Build history of the part. All positions in model axes, mm. A direction names the side the tool comes from. Give positions to 0.01 mm unless a question says otherwise; leave off trailing zeros. Order: outer loops, then holes, each group sorted by start corner. A loop starts at its lowest first (then second) coordinate and runs counter-clockwise, first axis right, second up. Notation, with made-up numbers: M 22.5,0.5 L 69.5,0.5 A17 ccw 69.5,8.5 Z; hole C 86.5,-35 d2. An arc over 180 degrees is marked long. Answer as CSV lines item,"result".
from build123d import *

# Parameters (mm, degrees)
SKETCH_1_R      = 1.75
SKETCH_1_W      = 65.5
SKETCH_1_H      = 80
EXTRUDE_1_DEPTH = 1
FILLET_1_R      = 1
FILLET_2_R      = 2


with BuildPart() as part:
    # 草圖1 → 填料-伸長1 (new body)
    with BuildSketch(Plane.XY):
        Polygon((-35.75, -20.56252042), (-43, -20.56252042), (-43, -50), (-25.75, -50), (25.75, -50), (43, -50), (43, -20.56252042), (35.75, -20.56252042), (35.75, 20.56252042), (43, 20.56252042), (43, 50), (25.75, 50), (-25.75, 50), (-43, 50), (-43, 20.56252042), (-35.75, 20.56252042), align=None)
        with Locations((-40, -26)):
            Circle(SKETCH_1_R, mode=Mode.SUBTRACT)
        with Locations(Location((40, -26, 0), (0, 0, 180))):
            Circle(SKETCH_1_R, mode=Mode.SUBTRACT)
        with Locations((40, 26)):
            Circle(SKETCH_1_R, mode=Mode.SUBTRACT)
        with Locations(Location((-40, 26, 0), (0, 0, 180))):
            Circle(SKETCH_1_R, mode=Mode.SUBTRACT)
        with Locations((-40, -46)):
            Circle(SKETCH_1_R, mode=Mode.SUBTRACT)
        with Locations(Location((-40, 46, 0), (0, 0, 180))):
            Circle(SKETCH_1_R, mode=Mode.SUBTRACT)
        with Locations((40, 46)):
            Circle(SKETCH_1_R, mode=Mode.SUBTRACT)
        with Locations(Location((40, -46, 0), (0, 0, 180))):
            Circle(SKETCH_1_R, mode=Mode.SUBTRACT)
        Rectangle(SKETCH_1_W, SKETCH_1_H, mode=Mode.SUBTRACT)
        with BuildLine():
            Line((-22, -43), (-11, -43))
            ThreePointArc((-11, -43), (-9, -45), (-11, -47))
            Line((-11, -47), (-22, -47))
            ThreePointArc((-22, -47), (-24, -45), (-22, -43))
        make_face(mode=Mode.SUBTRACT)
        with BuildLine():
            Line((22, -43), (11, -43))
            ThreePointArc((11, -43), (9, -45), (11, -47))
            Line((11, -47), (22, -47))
            ThreePointArc((22, -47), (24, -45), (22, -43))
        make_face(mode=Mode.SUBTRACT)
        with BuildLine():
            Line((22, 43), (11, 43))
            ThreePointArc((11, 43), (9, 45), (11, 47))
            Line((11, 47), (22, 47))
            ThreePointArc((22, 47), (24, 45), (22, 43))
        make_face(mode=Mode.SUBTRACT)
        with BuildLine():
            Line((-22, 43), (-11, 43))
            ThreePointArc((-11, 43), (-9, 45), (-11, 47))
            Line((-11, 47), (-22, 47))
            ThreePointArc((-22, 47), (-24, 45), (-22, 43))
        make_face(mode=Mode.SUBTRACT)
    extrude(amount=EXTRUDE_1_DEPTH)

    # 圓角1
    fillet_1_edges = [part.edges().sort_by_distance(p)[0] for p in [
        (35.75, 20.56252042, 0.5),
        (35.75, -20.56252042, 0.5),
        (-35.75, -20.56252042, 0.5),
        (-35.75, 20.56252042, 0.5),
    ]]
    fillet(fillet_1_edges, radius=FILLET_1_R)

    # 圓角2
    fillet_2_edges = [part.edges().sort_by_distance(p)[0] for p in [
        (43, 50, 0.5),
        (43, 20.56252042, 0.5),
        (43, -20.56252042, 0.5),
        (43, -50, 0.5),
        (-43, -50, 0.5),
        (-43, -20.56252042, 0.5),
        (-43, 20.56252042, 0.5),
        (-43, 50, 0.5),
    ]]
    fillet(fillet_2_edges, radius=FILLET_2_R)


solid = part.part
Item 1: 3-axis set-ups, long thin cutter, end or side, ignore diameter. For faces 1 (the flat face through (35, 4, 0)), 2 (the cylindrical face through (42.43, 21.164, 0.507)), 3 (the cylindrical face through (9, 45, 0.5)): which of +Z, -Z, +X, -X, +Y, -Y reach the whole face in a straight line?
Geometry says:
face 1,"-Z, +X, -X, +Y, -Y"
face 2,"+Z, -Z, +X"
face 3,"+Z, -Z"
Item 2: Band-saw the part on A-A (y = 26). Give the cut face in (x, z), and give its area (3 significant figures).
Geometry says:
outline,"M -43,0 L -41.75,0 L -41.75,1 L -43,1 Z; M -38.25,0 L -32.75,0 L -32.75,1 L -38.25,1 Z; M 32.75,0 L 38.25,0 L 38.25,1 L 32.75,1 Z; M 41.75,0 L 43,0 L 43,1 L 41.75,1 Z"
area,"13.5 mm2"
Item 3: Probe line 1 along Y through (x, z) = (-21, 0.65); line 2 along Y through (x, z) = (-40, 0.8); line 3 along Y through (x, z) = (7.5, 0.85). List the from-to ranges inside material, lowest first. Write a range as from..to.
Geometry says:
line 1,"y = -50..-47, -43..-40, 40..43, 47..50"
line 2,"y = -50..-47.75, -44.25..-27.75, -24.25..-20.56, 20.56..24.25, 27.75..44.25, 47.75..50"
line 3,"y = -50..-40, 40..50"
Item 4: Band-saw the part on D-D (y = -11). Give the cut face in (x, z).
Geometry says:
outline,"M -35.75,0 L -32.75,0 L -32.75,1 L -35.75,1 Z; M 32.75,0 L 35.75,0 L 35.75,1 L 32.75,1 Z"
Item 5: Band-saw the part on C-C (x = 17). Give the cut face in (y, z).
Geometry says:
outline,"M -50,0 L -47,0 L -47,1 L -50,1 Z; M -43,0 L -40,0 L -40,1 L -43,1 Z; M 40,0 L 43,0 L 43,1 L 40,1 Z; M 47,0 L 50,0 L 50,1 L 47,1 Z"
Item 6: Drop a flat-ended pin along its axis: pin 1 (0.5 mm diameter, centred on y = -7, z = 0.5, fed in from +X). Give the stop position or say it passes through.
Geometry says:
pin 1,"stops at x = 35.75"
Item 7: Pull direction X, two halves, no side cores. Call faces 4 (the cylindrical face through (-9, 45, 0.5)), 5 (the cylindrical face through (42.4, -49.43, 0.51)), 6 (the cylindrical face through (-42.399, 21.133, 0.507)): released by +X, released by -X, zero draft, split by the parting line, or undercut.
Geometry says:
face 4,"undercut"
face 5,"released by +X"
face 6,"released by -X"
Item 8: Band-saw the part on B-B (x = 2). Give the cut face in (y, z), and give its area (3 significant figures).
Geometry says:
outline,"M -50,0 L -40,0 L -40,1 L -50,1 Z; M 40,0 L 50,0 L 50,1 L 40,1 Z"
area,"20.0 mm2"
